Could you check a few things on this drawing? It's one solid part, dimensions in mm from its lowest x, y, z. Round coordinates to 2 decimals unless told otherwise and drop trailing zeros. Loops run counter-clockwise (first coordinate to the right, second up) from the corner with the lowest first, then second, coordinate; pieces in that order, holes last. Notation, with made-up numbers: (71.25, -14) -> (115.25, -14) arc R25 cw to (115.25, 20) -> close; hole circle Ø6 at (84.5, -36). An arc over 180 degrees is marked (long way). Use one line per item in the form item = value. Start each with the question number.
Item 1: If we section it at A-A (z = 51): Write out the boundary of the cut face in (x, y) (3 decimals), then the cut area to 3 significant figures.
Item 2: If I drill on L1, parallel to Y at x = 5, z = 24.5; L2, parallel to X at y = 7.75, z = 55.5, over which ranges is the centre line in solid material (lowest first)? Write a range as [from, to].
Item 3: I'm going to push flat-ended pins straight in: pin 1 Ø1 at (x, z) = (2.5, 40) entering from +Y; pin 2 Ø5 at (y, z) = (1, 50.5) entering from +X; pin 3 Ø1 at (x, z) = (4, 20.5) entering from +Y. Where does each tip first touch, or does it pass through?
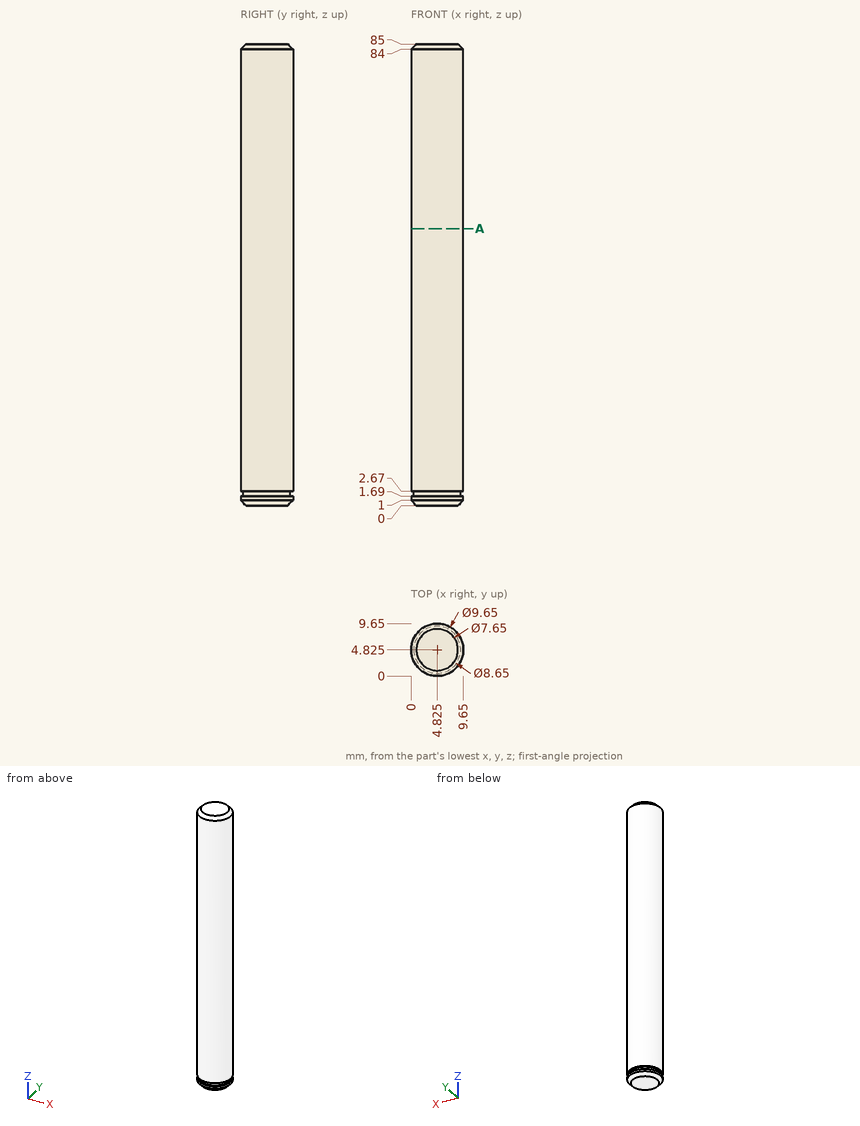
Values found:
q1.outline = circle Ø9.65 at (4.825, 4.825)
q1.area = 73.1 mm2
q2.L1 = [0, 9.65]
q2.L2 = [0.99, 8.66]
q3.pin_1 = 9.29
q3.pin_2 = 9.46
q3.pin_3 = 9.64
